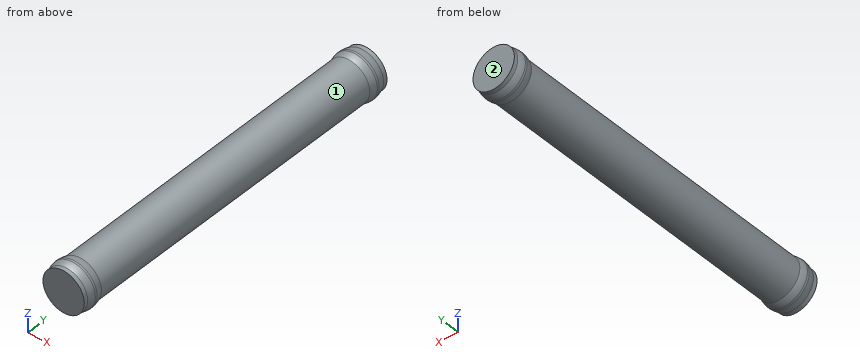
```python
from build123d import *

# Parameters (mm, degrees)
F0_R     = 3.302
F1_DEPTH = 55.88
F3_R     = 3.556
F4_DEPTH = 1.27


# Not quite as in the source:
# - a fillet or chamfer that OpenCascade refuses, or shapes differently, is made with other operations: its cross-section is extruded or revolved along the edge and cut away or added
# - a feature names something its author has since deleted; it is built from what else it names


with BuildPart() as f1:
    # F0 (on Front) → F1 (new body)
    with BuildSketch(Plane.XZ):
        with Locations((-16.002, 0)):
            Circle(F0_R)
    extrude(amount=F1_DEPTH)

    # F3 (on offset) → F4 (join, symmetric)
    with BuildSketch(Plane.XZ.offset(53.975)):
        with Locations((-16.002, 0)):
            Circle(F3_R)
    extrude(amount=F4_DEPTH, both=True)

    # F6: F1 across plane


with BuildPart() as f1_1:
    add(f1.part)
    add(f1.part.mirror(Plane(origin=(-16.002, -27.94, 0), x_dir=(1, 0, 0), z_dir=(0, -1, 0))))

    # F7: fillet of radius 2.54 on 4 edges, made by hand

    # F7_s1 → F7_t2 (revolve, cut)
    with BuildSketch(Plane.XY):
        with BuildLine():
            ThreePointArc((-12.446, -54.1378396683), (-12.5103142364, -54.7058009346), (-12.7, -55.245))
            Line((-12.7, -55.245), (-12.446, -55.245))
            Line((-12.446, -55.245), (-12.446, -54.1378396683))
        make_face()
    revolve(axis=Axis((-16.002, -55.245, 0), (0, -1, 0)), mode=Mode.SUBTRACT)

    # F7_s3 → F7_t4 (revolve, cut)
    with BuildSketch(Plane.XY):
        with BuildLine():
            ThreePointArc((-12.7, -52.705), (-12.5103142364, -53.2441990654), (-12.446, -53.8121603317))
            Line((-12.446, -53.8121603317), (-12.446, -52.705))
            Line((-12.446, -52.705), (-12.7, -52.705))
        make_face()
    revolve(axis=Axis((-16.002, -52.705, 0), (0, -1, 0)), mode=Mode.SUBTRACT)

    # F7_s5 → F7_t6 (revolve, cut)
    with BuildSketch(Plane.XY):
        with BuildLine():
            ThreePointArc((-12.446, -2.0678396683), (-12.5103142364, -2.6358009346), (-12.7, -3.175))
            Line((-12.7, -3.175), (-12.446, -3.175))
            Line((-12.446, -3.175), (-12.446, -2.0678396683))
        make_face()
    revolve(axis=Axis((-16.002, -3.175, 0), (0, -1, 0)), mode=Mode.SUBTRACT)

    # F7_s7 → F7_t8 (revolve, cut)
    with BuildSketch(Plane.XY):
        with BuildLine():
            ThreePointArc((-12.7, -0.635), (-12.5103142364, -1.1741990654), (-12.446, -1.7421603317))
            Line((-12.446, -1.7421603317), (-12.446, -0.635))
            Line((-12.446, -0.635), (-12.7, -0.635))
        make_face()
    revolve(axis=Axis((-16.002, -0.635, 0), (0, -1, 0)), mode=Mode.SUBTRACT)


solid = f1_1.part
```
Read the model definition and answer for the solid it produces. Units are mm, in the model's axes. Face numbers are marked on the shaded views. A direction names the side the tool comes from. Round coordinates to 2 decimals unless told otherwise and drop trailing zeros. Write each loop counter-clockwise with the first axis right and the second up, starting at its lowest first coordinate (ties: lowest second). Pieces come first, ordered by that corner, then holes. Notation, with made-up numbers: M 50,-11 L 93,-11 A5 cw 93,-3 Z; hole C -10,58.5 d4. An arc over 180 degrees is marked long. One line per item, written item: value.
Q1. Straight lines are drawn through the part: line 1 (X direction, y = -24.5, z = 0); line 2 (Z direction, x = -14, y = -7); line 3 (Z direction, x = -15.5, y = -14.5). For each, find the intervals that lie inside material, in ascending order. Write a range as [from, to].
Data:
line 1: [-19.3, -12.7]
line 2: [-2.63, 2.63]
line 3: [-3.26, 3.26]
Q2. Find section A-A on y = -44. Write down the section's boundary in (x, z).
Data:
outline: C -16,0 d6.6
Q3. Which of the six approach directions +Z, -Z, +X, -X, +Y, -Y give full straight-line access (tool end or side, diameter ignored) to the marked faces 1 and 2?
Data:
face 1: none
face 2: +Z, -Z, +X, -X, +Y
Q4. Flat-ended cylindrical pins translate along their axes: pin 1 Ø1.5 at (x, y) = (-18.5, -48) entering from +Z; pin 2 Ø2 at (x, y) = (-17.5, -32.5) entering from -Z; pin 3 Ø3 at (y, z) = (-8, 1.5) entering from -X. Find the tip coordinate at first contact, or state that the pin passes through.
Data:
pin 1: z = 2.8
pin 2: z = -3.26
pin 3: x = -19.3
